Geometry: final body of the model. Coordinates: model frame, mm. A direction names the side the tool comes from. Coordinates: 2 decimals unless noted, no trailing zeros. Order: outer loops, then holes, each group sorted by start corner. A loop starts at its lowest first (then second) coordinate and runs counter-clockwise, first axis right, second up. Notation, with made-up numbers: (44, 66) -> (101, 66) arc R12 ccw to (101, 85) -> close; hole circle Ø1 at (59, -11). An arc over 180 degrees is marked (long way). Answer in a Markdown table with one row per item. Add a question column.
1) Section query B-B on y = 9.5. Return the cut outline in (x, z), then the cut area to 3 significant figures.
2) Section query A-A on z = 0. Return the cut outline in (x, y) (3 decimals), then the cut area to 3 significant figures.
3) Ray query, line 1 (Z direction, x = -0.25, y = 17.5); line 2 (Y direction, x = -1.25, z = -3) (3 decimals); line 3 (X direction, y = 24, z = 2.5). Return the intervals inside material, ascending. Write a range as from..to.
4) Section query C-C on x = 0. Return the cut outline in (y, z) (3 decimals), then the cut area to 3 significant figures.
5) Section query D-D on y = 22. Return the cut outline in (x, z), then the cut area to 3 significant figures.
6) Contact query for flat-ended pins moving along their axis: P1, Ø1.5, axis at x = 1, y = 8, coming from the -Z side; P2, Ø6, axis at y = 2.5, z = 4.5, coming from the +X side; P3, Ø3, axis at x = 1.5, y = 20.5, coming from the +Z side; P4, Ø1.5, axis at x = 4, z = 2, coming from the -Y side (3 decimals). Output: stop coordinate, or through.
7) Set-up query: faces 1 (the face through (0, 0, 0)), 2 (the face through (-3.755, 16.277, 4.095)). Return all of +Z, -Z, +X, -X, +Y, -Y with unobstructed straight access to the full face (end or side cutting, diameter ignored); none if empty.
```python
from build123d import *

# Parameters (mm, degrees)
FILLET1_R = 0.508


with BuildPart() as part:
    # Sketch1 → Revolve1 (revolve)
    with BuildSketch(Plane.XY, mode=Mode.PRIVATE) as revolve1_sk:
        Polygon((0, 0), (2.38125, 0), (2.38125, 6.35), (2.12725, 6.604), (2.38125, 6.858), (2.38125, 15.875), (5.55625, 15.875), (5.55625, 16.66875), (6.35, 16.66875), (6.35, 26.19375), (0, 26.19375), align=None)
    revolve(revolve1_sk.sketch.rotate(Axis((0, 0, 0), (0, 1, 0)), 90), axis=Axis((0, 0, 0), (0, 1, 0)))  # turned: the seam where the file's is

    # Fillet1
    fillet1_edges = [part.edges().sort_by_distance(p)[0] for p in [
        (0, 26.19375, 6.35),
        (0, 16.66875, 6.35),
    ]]
    fillet(fillet1_edges, radius=FILLET1_R)


solid = part.part
```
Result:
| question | item | result |
|---|---|---|
| 1 | outline | circle Ø4.76 at (0, 0) |
| 1 | area | 17.8 mm2 |
| 2 | outline | (-6.35, 17.177) arc R0.508 ccw to (-5.842, 16.669) -> (-5.556, 16.669) -> (-5.556, 15.875) -> (-2.381, 15.875) -> (-2.381, 6.858) -> (-2.127, 6.604) -> (-2.381, 6.35) -> (-2.381, 0) -> (2.381, 0) -> (2.381, 6.35) -> (2.127, 6.604) -> (2.381, 6.858) -> (2.381, 15.875) -> (5.556, 15.875) -> (5.556, 16.669) -> (5.842, 16.669) arc R0.508 ccw to (6.35, 17.177) -> (6.35, 25.686) arc R0.508 ccw to (5.842, 26.194) -> (-5.842, 26.194) arc R0.508 ccw to (-6.35, 25.686) -> close |
| 2 | area | 205 mm2 |
| 3 | line 1 | -6.35..6.35 |
| 3 | line 2 | 15.875..26.194 |
| 3 | line 3 | -5.84..5.84 |
| 4 | outline | (0, -2.381) -> (6.35, -2.381) -> (6.604, -2.127) -> (6.858, -2.381) -> (15.875, -2.381) -> (15.875, -5.556) -> (16.669, -5.556) -> (16.669, -5.842) arc R0.508 ccw to (17.177, -6.35) -> (25.686, -6.35) arc R0.508 ccw to (26.194, -5.842) -> (26.194, 5.842) arc R0.508 ccw to (25.686, 6.35) -> (17.177, 6.35) arc R0.508 ccw to (16.669, 5.842) -> (16.669, 5.556) -> (15.875, 5.556) -> (15.875, 2.381) -> (6.858, 2.381) -> (6.604, 2.127) -> (6.35, 2.381) -> (0, 2.381) -> close |
| 4 | area | 205 mm2 |
| 5 | outline | circle Ø12.7 at (0, 0) |
| 5 | area | 127 mm2 |
| 6 | P1 | z = -2.37 |
| 6 | P2 | x = 1.85 |
| 6 | P3 | z = 6.35 |
| 6 | P4 | y = 15.875 |
| 7 | face 1 | +Z, -Z, +X, -X, -Y |
| 7 | face 2 | -Y |
